Part model, mm, in its own coordinate system. A direction names the side the tool comes from. Coordinates: 2 decimals unless noted, no trailing zeros. Loops run counter-clockwise (first coordinate to the right, second up) from the corner with the lowest first, then second, coordinate; pieces in that order, holes last. Notation, with made-up numbers: M -5,75 L 30,75 A27 cw 30,93 Z; hole C -5,65.5 d10. An arc over 180 degrees is marked long. Answer as a JSON object with one key per item and string values. Group by question number.
1. Saw through at C-C on x = 57. Write the cut outline in (y, z) (3 decimals).
2. Drop flat-ended pins along their axis: pin 1 Ø6 at (y, z) = (3, 7.5) entering from -X; pin 2 Ø10 at (x, z) = (42.5, 0.5) entering from +Y (3 decimals); pin 3 Ø6 at (x, z) = (148, 1) entering from -Y (3 decimals). Give the stop position or say it passes through.
3. Drill centre lines: L1, parallel to X at y = 0.5, z = -4.5; L2, parallel to Y at x = 232.5, z = -0.25; L3, parallel to Y at x = 152.5, z = -1.25. Where is each one in solid material? Low to high.
4. Mould opens along X. For faces 3 (the face through (265.125, 0, 0)), 4 (the face through (123.55, -0.69, -3.1)), 5 (the face through (243.688, 4, 0)) say: released by +X, released by -X, zero draft, split by the parting line, or undercut.
5. 3-axis set-ups, long thin cutter, end or side, ignore diameter. For faces 1 (the face through (-6.12, -0.69, -3.1)), 2 (the face through (-12.7, 0, 0)): which of +Z, -Z, +X, -X, +Y, -Y reach the whole face in a straight line?
6. Saw through at A-A on z = 0. Write the cut outline in (x, y) (3 decimals).
Autodesk Inventor part; units mm, degrees
ref_plane "rod_cp_XY" through (0, 0, 0) normal (1, 0, 0) x (0, 0, -1)
ref_plane "rod_cp_YZ" through (0, 0, 0) normal (0, 0, -1) x (0, 1, 0)
ref_plane "rod_cp_ZX" through (0, 0, 0) normal (0, 1, 0) x (1, 0, 0)
sketch "Sketch_1" plane through (0, 0, 0) normal (0, 0, 1) x (1, 0, 0)
  line L0 (265.1252, 0) -> (0, 0)
  line L1 (0, 0) -> (0, 3.175)
  line L2 (0, 3.175) -> (243.6876, 3.175)
  line L3 (243.6876, 3.175) -> (243.6876, 9.6203)
  line L4 (243.6876, 9.6203) -> (265.1252, 9.6203)
  line L5 (265.1252, 9.6203) -> (265.1252, 0)
  line L6 (265.1252, 0) -> (0, 0)
revolve "Revolution1" add sketch "Sketch_1" angle 360 about axis through (265.1252, 0, 0) along (1, 0, 0)
sketch "Sketch_3" plane through (0, 0, 0) normal (0, 0, 1) x (1, 0, 0)
  line L0 (0, 0) -> (-12.7, 0)
  line L1 (-12.7, 0) -> (-12.7, 2.634)
  line L2 (-12.7, 2.634) -> (-12.159, 3.175)
  line L3 (-12.159, 3.175) -> (0, 3.175)
  line L4 (0, 3.175) -> (0, 0)
  line L5 (0, 0) -> (-12.7, 0)
revolve "Revolution2" add sketch "Sketch_3" angle 360 about axis through (0, 0, 0) along (1, 0, 0)
thread "Thread1"
sketch "Sketch_30" plane through (0, 0, 0) normal (0, 0, 1) x (1, 0, 0)
  line L0 (0, 0) -> (-0.254, 0)
  line L1 (-0.254, 3.429) -> (-0.254, 2.921)
  line L2 (-0.254, 2.921) -> (0, 2.921)
  line L3 (0, 2.921) -> (0, 3.429)
  line L4 (0, 3.429) -> (-0.254, 3.429)
revolve "Revolution3" cut sketch "Sketch_30" angle 360 about axis through (0, 0, 0) along (1, 0, 0)
ref_plane "rod_cp_XY" through (0, 0, 0) normal (1, 0, 0) x (0, 0, -1)
ref_plane "rod_cp_YZ" through (0, 0, 0) normal (0, 0, -1) x (0, 1, 0)
ref_plane "rod_cp_ZX" through (0, 0, 0) normal (0, 1, 0) x (1, 0, 0)
ref_plane "to_rod_clevis_XY" through (-12.7, 0, 0) normal (1, 0, 0) x (0, 0, -1)
ref_plane "to_rod_clevis_YZ" through (-12.7, 0, 0) normal (0, 0, -1) x (0, 1, 0)
ref_plane "to_rod_clevis_ZX" through (-12.7, 0, 0) normal (0, 1, 0) x (1, 0, 0)
ref_plane "rl2_XY" through (0, 0, 0) normal (1, 0, 0) x (0, 0, -1)
ref_plane "rl2_YZ" through (0, 0, 0) normal (0, 0, -1) x (0, 1, 0)
ref_plane "rl2_ZX" through (0, 0, 0) normal (0, 1, 0) x (1, 0, 0)
ref_plane "rl1_XY" through (-12.7, 0, 0) normal (1, 0, 0) x (0, 0, -1)
ref_plane "rl1_YZ" through (-12.7, 0, 0) normal (0, 0, -1) x (0, 1, 0)
ref_plane "rl1_ZX" through (-12.7, 0, 0) normal (0, 1, 0) x (1, 0, 0)
ref_plane "thd1_XY" through (-12.7, 3.175, 0) normal (1, 0, 0) x (0, 0, -1)
ref_plane "thd1_YZ" through (-12.7, 3.175, 0) normal (0, 0, -1) x (0, 1, 0)
ref_plane "thd1_ZX" through (-12.7, 3.175, 0) normal (0, 1, 0) x (1, 0, 0)
ref_plane "thd2_XY" through (-12.7, -3.175, 0) normal (1, 0, 0) x (0, 0, -1)
ref_plane "thd2_YZ" through (-12.7, -3.175, 0) normal (0, 0, -1) x (0, 1, 0)
ref_plane "thd2_ZX" through (-12.7, -3.175, 0) normal (0, 1, 0) x (1, 0, 0)
ref_plane "dia1_XY" through (0, 3.175, 0) normal (1, 0, 0) x (0, 0, -1)
ref_plane "dia1_YZ" through (0, 3.175, 0) normal (0, 0, -1) x (0, 1, 0)
ref_plane "dia1_ZX" through (0, 3.175, 0) normal (0, 1, 0) x (1, 0, 0)
ref_plane "dia2_XY" through (0, -3.175, 0) normal (1, 0, 0) x (0, 0, -1)
ref_plane "dia2_YZ" through (0, -3.175, 0) normal (0, 0, -1) x (0, 1, 0)
ref_plane "dia2_ZX" through (0, -3.175, 0) normal (0, 1, 0) x (1, 0, 0)
ref_plane "hh1_XY" through (295.2496, 0, 0) normal (0, 0, 1) x (1, 0, 0)
ref_plane "hh1_YZ" through (295.2496, 0, 0) normal (1, 0, 0) x (0, 1, 0)
ref_plane "hh1_ZX" through (295.2496, 0, 0) normal (0, 1, 0) x (0, 0, 1)
ref_plane "hh2_XY" through (301.6504, 0, 0) normal (0, 0, 1) x (1, 0, 0)
ref_plane "hh2_YZ" through (301.6504, 0, 0) normal (1, 0, 0) x (0, 1, 0)
ref_plane "hh2_ZX" through (301.6504, 0, 0) normal (0, 1, 0) x (0, 0, 1)
ref_plane "dia12_XY" through (0, 0, 10.9537) normal (1, 0, 0) x (0, 0, -1)
ref_plane "dia12_YZ" through (0, 0, 10.9537) normal (0, 0, -1) x (0, 1, 0)
ref_plane "dia12_ZX" through (0, 0, 10.9537) normal (0, 1, 0) x (1, 0, 0)
ref_plane "dia22_XY" through (0, 0, -10.9537) normal (1, 0, 0) x (0, 0, -1)
ref_plane "dia22_YZ" through (0, 0, -10.9537) normal (0, 0, -1) x (0, 1, 0)
ref_plane "dia22_ZX" through (0, 0, -10.9537) normal (0, 1, 0) x (1, 0, 0)
properties part number "048-DXP0_rod"
Outcome:
{
 "1": {"outline": "C 0,0 d6.35"},
 "2": {"pin 1": "stops at x = 243.69", "pin 2": "stops at y = 3.175", "pin 3": "stops at y = -3.175"},
 "3": {"L1": "x = 243.69 to 265.13", "L2": "y = -3.17 to 3.17", "L3": "y = -2.92 to 2.92"},
 "4": {"face 3": "released by +X", "face 4": "zero draft", "face 5": "released by -X"},
 "5": {"face 1": "-X", "face 2": "+Z, -Z, -X, +Y, -Y"},
 "6": {"outline": "M -12.7,-2.634 L -12.159,-3.175 L -0.254,-3.175 L -0.254,-2.921 L 0,-2.921 L 0,-3.175 L 243.688,-3.175 L 243.688,-9.62 L 265.125,-9.62 L 265.125,9.62 L 243.688,9.62 L 243.688,3.175 L 0,3.175 L 0,2.921 L -0.254,2.921 L -0.254,3.175 L -12.159,3.175 L -12.7,2.634 Z"}
}
